```python
from build123d import *

# Parameters (mm, degrees)
EXTRUDE_1_DEPTH               = 9
CUT_EXTRUDE_1_DEPTH           = 30.816103032
CUT_EXTRUDE_1_DEPTH_BACK      = 30.816103032
SKETCH_2_R                    = 2.3
CUT_EXTRUDE_2_DEPTH           = 3.3
CUT_EXTRUDE_2_OTHER_WAY_DEPTH = 36.043722716
CUT_EXTRUDE_2_OTHER_WAY_TAPER = 1
CUT_EXTRUDE_3_DEPTH           = 36.043722716
CUT_EXTRUDE_3_DEPTH_BACK      = 4
CUT_EXTRUDE_4_REACH           = 46.777
CUT_EXTRUDE_4_END_RADIUS      = 10.2
SKETCH_5_R                    = 1.6
SKETCH_6_R                    = 2.2
CUT_EXTRUDE_5_DEPTH           = 30.816103062
CUT_EXTRUDE_START             = -5.5
SKETCH_7_R                    = 4
SKETCH_7_R_2                  = 2.2
CUT_EXTRUDE_6_DEPTH           = 5.5


with BuildPart() as part:
    # Эскиз1 → Бобышка-Вытянуть1 (new, symmetric)
    with BuildSketch(Plane(origin=(0, 0, 0), x_dir=(0, 0, -1), z_dir=(1, 0, 0))):
        with BuildLine():
            Line((-0.75, -21), (-0.75, -11.06243644))
            ThreePointArc((-0.75, -11.06243644), (-0.989654684, -10.412917388), (-1.59375, -10.074718901))
            ThreePointArc((-1.59375, -10.074718901), (0, 10.2), (1.59375, -10.074718901))
            ThreePointArc((1.59375, -10.074718901), (0.989654684, -10.412917388), (0.75, -11.06243644))
            Line((0.75, -11.06243644), (0.75, -21))
            ThreePointArc((0.75, -21), (1.042893219, -21.707106781), (1.75, -22))
            Line((1.75, -22), (6.75, -22))
            ThreePointArc((6.75, -22), (7.457106781, -21.707106781), (7.75, -21))
            Line((7.75, -21), (7.75, -13.898830886))
            ThreePointArc((7.75, -13.898830886), (8.121662204, -12.215036114), (9.167582418, -10.844142779))
            ThreePointArc((9.167582418, -10.844142779), (13.897042702, -2.917568189), (12.75462481, 6.241758242))
            ThreePointArc((12.75462481, 6.241758242), (12.953882386, 10.117431577), (16.34747687, 12))
            Line((16.34747687, 12), (17, 12))
            ThreePointArc((17, 12), (17.707106781, 12.292893219), (18, 13))
            Line((18, 13), (18, 18))
            Line((18, 18), (-18, 18))
            Line((-18, 18), (-18, 13))
            ThreePointArc((-18, 13), (-17.707106781, 12.292893219), (-17, 12))
            Line((-17, 12), (-16.34747687, 12))
            ThreePointArc((-16.34747687, 12), (-12.953882386, 10.117431577), (-12.75462481, 6.241758242))
            ThreePointArc((-12.75462481, 6.241758242), (-13.897042702, -2.917568189), (-9.167582418, -10.844142779))
            ThreePointArc((-9.167582418, -10.844142779), (-8.121662204, -12.215036114), (-7.75, -13.898830886))
            Line((-7.75, -13.898830886), (-7.75, -21))
            ThreePointArc((-7.75, -21), (-7.457106781, -21.707106781), (-6.75, -22))
            Line((-6.75, -22), (-1.75, -22))
            ThreePointArc((-1.75, -22), (-1.042893219, -21.707106781), (-0.75, -21))
        make_face()
    extrude(amount=EXTRUDE_1_DEPTH, both=True)

    # Эскиз2 → Вырез-Вытянуть1 (cut, two sides: drawn at the far end of the back side and taken through both)
    with BuildSketch(Plane.XY.offset(-CUT_EXTRUDE_1_DEPTH_BACK)):
        with BuildLine():
            ThreePointArc((-3.1, 18), (0, 14.9), (3.1, 18))
            Line((3.1, 18), (-3.1, 18))
        make_face()
        with Locations(Location((0, -16, 0), (0, 0, 66.000891847))):
            Circle(SKETCH_2_R)
    extrude(amount=CUT_EXTRUDE_1_DEPTH + CUT_EXTRUDE_1_DEPTH_BACK, mode=Mode.SUBTRACT)

    # Эскиз3 → Вырез-Вытянуть2 (cut)
    with BuildSketch(Plane(origin=(0, 0, -7.75), x_dir=(-1, 0, 0), z_dir=(0, 0, -1))):
        Polygon((-4.618802154, -16), (-2.309401077, -20), (2.309401077, -20), (4.618802154, -16), (2.309401077, -12), (-2.309401077, -12), align=None)
    extrude(amount=-CUT_EXTRUDE_2_DEPTH, mode=Mode.SUBTRACT)

    # Эскиз3 → Вырез-Вытянуть2 other way (cut)
    with BuildSketch(Plane(origin=(0, 0, -7.75), x_dir=(-1, 0, 0), z_dir=(0, 0, -1))):
        Polygon((-4.618802154, -16), (-2.309401077, -20), (2.309401077, -20), (4.618802154, -16), (2.309401077, -12), (-2.309401077, -12), align=None)
    extrude(amount=CUT_EXTRUDE_2_OTHER_WAY_DEPTH, taper=CUT_EXTRUDE_2_OTHER_WAY_TAPER, mode=Mode.SUBTRACT)

    # Эскиз4 → Вырез-Вытянуть3 (cut, two sides: drawn at the far end of the back side and taken through both)
    with BuildSketch(Plane.XY.offset(7.75).offset(-CUT_EXTRUDE_3_DEPTH_BACK)):
        with BuildLine():
            Line((-3.403687464, -13.898830886), (-0.935461573, -13.898830886))
            ThreePointArc((-0.935461573, -13.898830886), (0, -18.3), (0.935461573, -13.898830886))
            Line((0.935461573, -13.898830886), (3.403687464, -13.898830886))
            ThreePointArc((3.403687464, -13.898830886), (0, -12), (-3.403687464, -13.898830886))
        make_face()
        with BuildLine():
            ThreePointArc((0.935461573, -13.898830886), (0, -18.3), (-0.935461573, -13.898830886))
            Line((-0.935461573, -13.898830886), (-3.403687464, -13.898830886))
            ThreePointArc((-3.403687464, -13.898830886), (-1.092073748, -19.848035204), (4, -16))
            ThreePointArc((4, -16), (3.848035204, -14.907926252), (3.403687464, -13.898830886))
            Line((3.403687464, -13.898830886), (0.935461573, -13.898830886))
        make_face()
        with BuildLine():
            Line((-3.403687464, -13.898830886), (-0.935461573, -13.898830886))
            ThreePointArc((-0.935461573, -13.898830886), (0, -18.3), (0.935461573, -13.898830886))
            Line((0.935461573, -13.898830886), (3.403687464, -13.898830886))
            ThreePointArc((3.403687464, -13.898830886), (0, -12), (-3.403687464, -13.898830886))
        make_face()
        with BuildLine():
            ThreePointArc((0.935461573, -13.898830886), (0, -18.3), (-0.935461573, -13.898830886))
            Line((-0.935461573, -13.898830886), (-3.403687464, -13.898830886))
            ThreePointArc((-3.403687464, -13.898830886), (-1.092073748, -19.848035204), (4, -16))
            ThreePointArc((4, -16), (3.848035204, -14.907926252), (3.403687464, -13.898830886))
            Line((3.403687464, -13.898830886), (0.935461573, -13.898830886))
        make_face()
    extrude(amount=CUT_EXTRUDE_3_DEPTH + CUT_EXTRUDE_3_DEPTH_BACK, mode=Mode.SUBTRACT)

    # Вырез-Вытянуть4: up to this cylinder (the profile starts outside it)
    cut_extrude_4_end = Plane(origin=(0, 0, 0), z_dir=(-1, 0, 0)) * Cylinder(CUT_EXTRUDE_4_END_RADIUS, 127.454, mode=Mode.PRIVATE)
    # Эскиз5 → Вырез-Вытянуть4 (cut, up to the surface)
    with BuildSketch(Plane(origin=(0, 18, 0), x_dir=(1, 0, 0), z_dir=(0, 1, 0)), mode=Mode.PRIVATE) as cut_extrude_4_sk1:
        with Locations(Location((6.25, 0, 0), (0, 0, 270))):
            Circle(SKETCH_5_R)
    cut_extrude_4_tool1 = extrude(cut_extrude_4_sk1.sketch, amount=-CUT_EXTRUDE_4_REACH, mode=Mode.PRIVATE) - cut_extrude_4_end
    add(cut_extrude_4_tool1.solids().sort_by_distance((6.25, 18, 0))[0], mode=Mode.SUBTRACT)
    # Эскиз5 → Вырез-Вытянуть4 (cut, up to the surface)
    with BuildSketch(Plane(origin=(0, 18, 0), x_dir=(1, 0, 0), z_dir=(0, 1, 0)), mode=Mode.PRIVATE) as cut_extrude_4_sk2:
        with Locations(Location((-6.25, 0, 0), (0, 0, 270))):
            Circle(SKETCH_5_R)
    cut_extrude_4_tool2 = extrude(cut_extrude_4_sk2.sketch, amount=-CUT_EXTRUDE_4_REACH, mode=Mode.PRIVATE) - cut_extrude_4_end
    add(cut_extrude_4_tool2.solids().sort_by_distance((-6.25, 18, 0))[0], mode=Mode.SUBTRACT)

    # Эскиз6 → Вырез-Вытянуть5 (cut, through all)
    with BuildSketch(Plane.XY):
        Circle(SKETCH_6_R)
    extrude(amount=-CUT_EXTRUDE_5_DEPTH, mode=Mode.SUBTRACT)

    # Эскиз7 → Вырез-Вытянуть6 (cut)
    with BuildSketch(Plane(origin=(0, 0, -18), x_dir=(-1, 0, 0), z_dir=(0, 0, -1)).offset(CUT_EXTRUDE_START)):
        Circle(SKETCH_7_R)
        with Locations(Location((0, 0, 0), (0, 0, 180))):
            Circle(SKETCH_7_R_2, mode=Mode.SUBTRACT)
    extrude(amount=CUT_EXTRUDE_6_DEPTH, mode=Mode.SUBTRACT)


solid = part.part
```
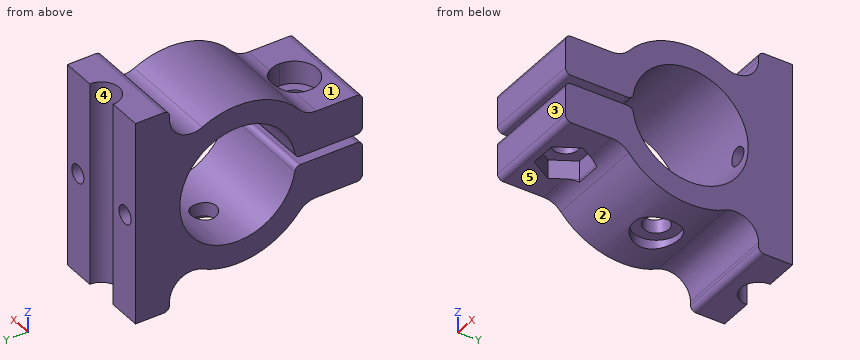
Input: part model. Units: mm. Frame: model coordinates. Face numbers are marked on the shaded views. A direction names the side the tool comes from. Coordinates: 2 decimals unless noted, no trailing zeros. Write each loop counter-clockwise with the first axis right and the second up, starting at its lowest first coordinate (ties: lowest second). Pieces come first, ordered by that corner, then holes. Notation, with made-up numbers: (-11.5, 54) - (37.5, 54) arc R27 ccw to (37.5, 76) - close; hole circle Ø9 at (71.25, 74.25). An arc over 180 degrees is marked (long way). Put each result on its own line as item: value. Start each with the question number.
1) Cut plane B-B (y = 0). Return the cut outline in (x, z), plus the area to 3 significant figures.
2) Reachability of the marked faces 4 and 5 from +Z, -Z, +X, -X, +Y, -Y: full face, straight path, thin tool, end or side. Return the list, or none.
3) Cut plane C-C (y = -4.5). Return the cut outline in (x, z).
4) Cut plane A-A (z = 0). Return the cut outline in (x, y).
5) Mould query, pull axis Y, two halves, no side actions, for the marked faces 1, 2 and 3. Classes: pulls with the +Y half, pulls with the -Y half, needs draft (parallel to the pull), parting line crosses it, or undercut.
6) Contact query for flat-ended pins moving along their axis: pin 1 (2.5 mm diameter, centred on x = 1.5, y = 1.5, fed in from -Z); pin 2 (3.5 mm diameter, centred on x = 6.25, z = 0, fed in from +Y); pin 3 (4 mm diameter, centred on x = 0, y = 0, fed in from -Z); pin 4 (3 mm diameter, centred on x = 7, y = -14.5, fed in from +Z). Output: stop coordinate, or through.
7) Ray query, L1, parallel to X at y = 12, z = 0; L2, parallel to Z at x = 6.25, y = 14.25; L3, parallel to X at y = -16, z = -1.95. Return the intervals inside material, ascending.
Resolved:
1. outline: (-9, -14.2) - (-4, -14.2) - (-4, -12.5) - (-2.2, -12.5) - (-2.2, -10.2) - (-9, -10.2) - close; (-9, 10.2) - (9, 10.2) - (9, 14.2) - (-9, 14.2) - close; (2.2, -12.5) - (4, -12.5) - (4, -14.2) - (9, -14.2) - (9, -10.2) - (2.2, -10.2) - close
1. area: 120 mm2
2. face 4: +Z, -Z, +Y
2. face 5: -Z, +X, -X, -Y
3. outline: (-9, -13.47) - (9, -13.47) - (9, -9.15) - (-9, -9.15) - close; (-9, 9.15) - (9, 9.15) - (9, 13.47) - (-9, 13.47) - close
4. outline: (-9, 10.2) - (-7.85, 10.2) - (-7.85, 18) - (-9, 18) - close; (-4.65, 10.2) - (4.65, 10.2) - (4.65, 18) - (3.1, 18) arc R3.1 cw to (-3.1, 18) - (-4.65, 18) - close; (7.85, 10.2) - (9, 10.2) - (9, 18) - (7.85, 18) - close
5. face 1: needs draft
5. face 2: undercut
5. face 3: pulls with the -Y half
6. pin 1: stops at z = -12.5
6. pin 2: stops at y = 18
6. pin 3: stops at z = 10
6. pin 4: stops at z = 7.85
7. L1: x = -9 to -7.85, -4.65 to 4.65, 7.85 to 9
7. L2: z = -18 to -1.6, 1.6 to 18
7. L3: x = -9 to -2.3, 2.3 to 9
